Can you work these out from the model? Positions are in its coordinate system, mm. A direction names the side the tool comes from. Round coordinates to 2 decimals unless told otherwise and drop trailing zeros. Write each loop counter-clockwise with the first axis right and the second up, starting at its lowest first coordinate (ties: lowest second). Pieces come first, ordered by that corner, then holes. Notation, with made-up numbers: M -17,43 L 28,43 A19 cw 28,51 Z; hole C 85,86 d8. An arc over 180 degrees is marked long. Answer as a JSON object with one key per item and string values. Group by question number.
1) On a 3-axis mill with a long thin cutter (end or side, diameter ignored), from which of +Z, -Z, +X, -X, +Y, -Y can I reach the whole of each face in a straight line? I mean faces 1 (the flat face through (55, 46, 0)), 2 (the flat face through (121.022, 33.037, 1.479)), 3 (the flat face through (-14.46, 34.89, 1.48)). Say none if no direction works.
2) Suppose I cut it at C-C, the plane x = 58. Write out the boundary of the cut face in (y, z), and give its area (3 significant figures).
3) I'm going to push flat-ended pins straight in: pin 1 Ø1.5 at (x, z) = (-10, 1.5) entering from +Y; pin 2 Ø7 at (x, y) = (5.94, 53.59) entering from +Z; pin 3 Ø1 at (y, z) = (38.5, 0.5) entering from -X. Where does each tip first touch, or does it pass through?
4) Suppose I cut it at B-B, the plane z = 2.2. State how many separate pieces and enclosed holes the cut face has, and give its area (3 significant figures).
5) Please list where these lines run through material, in increasing order: L1, parallel to Y at x = 14.5, z = 1.3; L2, parallel to X at y = 25, z = 1.25; L3, parallel to X at y = 30.5, z = 1.7. Write a range as [from, to].
6) Suppose I cut it at A-A, the plane x = 24. Write out the boundary of the cut face in (y, z).
Autodesk Inventor part; units mm, degrees
ref_plane "YZ Plane" through (0, 0, 0) normal (1, 0, 0) x (0, 1, 0)
ref_plane "XZ Plane" through (0, 0, 0) normal (0, 1, 0) x (-1, 0, 0)
ref_plane "XY Plane" through (0, 0, 0) normal (0, 0, 1) x (1, 0, 0)
sketch "スケッチ2" plane through (0, 0, 0) normal (0, 0, 1) x (1, 0, 0)
  circle A0 centre (127.6431, 30.2622) radius 1.5
  circle A1 centre (5.9362, 53.5882) radius 1.5
  line L0 (5.9362, 53.5882) -> (127.6431, 30.2622) construction
  circle A2 centre (5.9362, 53.5882) radius 4.025
  circle A3 centre (127.6431, 30.2622) radius 4.025
  arc A4 (127.2517, 23.2481) -> (128.9655, 37.1616) centre (127.6431, 30.2622) ccw
  line L1 (12.8357, 52.2659) -> (13.4004, 55.2122)
  line L2 (15.4628, 54.817) -> (26.0698, 52.7841)
  line L3 (28.1322, 52.3888) -> (27.5675, 49.4424)
  line L4 (14.8981, 51.8706) -> (25.5051, 49.8377)
  line L5 (120.7437, 31.5845) -> (121.3084, 34.5309)
  line L6 (119.246, 34.9262) -> (108.639, 36.9591)
  line L7 (106.5765, 37.3543) -> (106.0119, 34.408)
  line L8 (108.0743, 34.0127) -> (118.6813, 31.9798)
  circle A5 centre (19.3546, 46.4346) radius 3
  circle A6 centre (112.5307, 28.5767) radius 3
  line L9 (7.2586, 60.4876) -> (128.9655, 37.1616)
  arc A7 (17.9263, 42.1672) -> (21.5465, 42.5045) centre (19.3546, 46.4346) ccw
  arc A8 (109.041, 25.7356) -> (112.28, 24.0837) centre (112.5307, 28.5767) ccw
  line L10 (3.7066, 46.9264) -> (17.9263, 42.1672)
  line L11 (112.28, 24.0837) -> (127.2517, 23.2481)
  circle A9 centre (19.3546, 46.4346) radius 1.5
  circle A10 centre (112.5307, 28.5767) radius 1.5
  line L12 (32.3442, 48.5269) -> (21.5465, 42.5045)
  line L13 (109.041, 25.7356) -> (101.2351, 35.3235)
  line L14 (32.3442, 48.5269) -> (101.2351, 35.3235)
  arc A11 (108.639, 36.9591) -> (106.5765, 37.3543) centre (107.6078, 37.1567) ccw
  arc A12 (106.0119, 34.408) -> (108.0743, 34.0127) centre (107.0431, 34.2103) ccw
  arc A13 (121.3084, 34.5309) -> (119.246, 34.9262) centre (120.2772, 34.7285) ccw
  arc A14 (118.6813, 31.9798) -> (120.7437, 31.5845) centre (119.7125, 31.7821) ccw
  arc A15 (28.1322, 52.3888) -> (26.0698, 52.7841) centre (27.101, 52.5864) ccw
  arc A16 (25.5051, 49.8377) -> (27.5675, 49.4424) centre (26.5363, 49.64) ccw
  arc A17 (15.4628, 54.817) -> (13.4004, 55.2122) centre (14.4316, 55.0146) ccw
  arc A18 (12.8357, 52.2659) -> (14.8981, 51.8706) centre (13.8669, 52.0682) ccw
  line L15 (5.9362, 53.5882) -> (-32.8159, 25.1361) construction
  circle A19 centre (-32.8159, 25.1361) radius 1.5
  arc A20 (-34.5914, 27.5543) -> (-31.0404, 22.7179) centre (-32.8159, 25.1361) ccw
  line L16 (-34.5914, 27.5543) -> (-0.9595, 52.247)
  line L17 (-31.0404, 22.7179) -> (2.5914, 47.4106)
  arc A21 (7.2586, 60.4876) -> (-0.9595, 52.247) centre (5.9362, 53.5882) ccw
  arc A22 (2.5914, 47.4106) -> (3.7066, 46.9264) centre (5.9362, 53.5882) ccw
  point P0 (0, 0)
  point P1 (0, 0)
  dimension "d31" = 8.05
  dimension "d32" = 8.05
  dimension "d33" = 3
  dimension "d34" = 3
  dimension "d35" = 15
  dimension "d36" = 3
  dimension "d37" = 15
  dimension "d38" = 6
  dimension "d39" = 6
  dimension "d40" = 9
  dimension "d41" = 9
  dimension "d42" = 3
  dimension "d43" = 3
  dimension "d44" = 7.5
  dimension "d45" = 7.5
  dimension "d46" = 40
  dimension "d47" = 40
  dimension "d48" = 2.1
  dimension "d49" = 2.1
  dimension "d50" = 2.1
  dimension "d51" = 2.1
  dimension "d52" = 2.1
  dimension "d53" = 2.1
  dimension "d54" = 2.1
  dimension "d55" = 2.1
  dimension "d56" = 3
  dimension "d57" = 6
  dimension "d58" = 3
  dimension "d59" = 3
extrude "押し出し2" add sketch "スケッチ2" along normal blind 3 contours L11 A8 L13 L14 L12 A7 L10 A22 L17 A20 L16 A21 L9 A4 | A5 | A6
equation "\"d47\" = d46"
properties part number "台形サスバー"
Results:
{
 "1": {"face 1": "-Z, +X, -X, +Y, -Y", "face 2": "+Z, -Z", "face 3": "+Z, -Z, -Y"},
 "2": {"outline": "M 43.61,0 L 50.76,0 L 50.76,3 L 43.61,3 Z", "area": "21.5 mm^2"},
 "3": {"pin 1": "y = 46.16", "pin 2": "through", "pin 3": "x = -20.36"},
 "4": {"separate pieces": "1", "enclosed holes": "7", "area": "1,420 mm^2"},
 "5": {"L1": "[43.31, 51.23], [56.06, 59.1]", "L2": "[-35.81, -34.31], [-31.32, -27.93], [109.8, 132.3]", "L3": "[-30.58, -20.44], [105.16, 123.63], [131.66, 134.66]"},
 "6": {"outline": "M 43.87,0 L 50.13,0 L 50.13,3 L 43.87,3 Z; M 53.18,0 L 57.28,0 L 57.28,3 L 53.18,3 Z"}
}
